Answer from the drawing. Dimensions are ordinates in mm from the lowest x, y and z of the part. Round coordinates to 2 decimals unless told otherwise and drop trailing zeros. Loops run counter-clockwise (first coordinate to the right, second up) from the corner with the lowest first, then second, coordinate; pieces in that order, holes last. Notation, with made-up numbers: (9, 87.5) - (18, 87.5) arc R13 cw to (18, 111.5) - close; hole circle Ø11 at (42.25, 68.5). An arc over 180 degrees is marked (long way). Return JSON: item names as keys, results as strings.
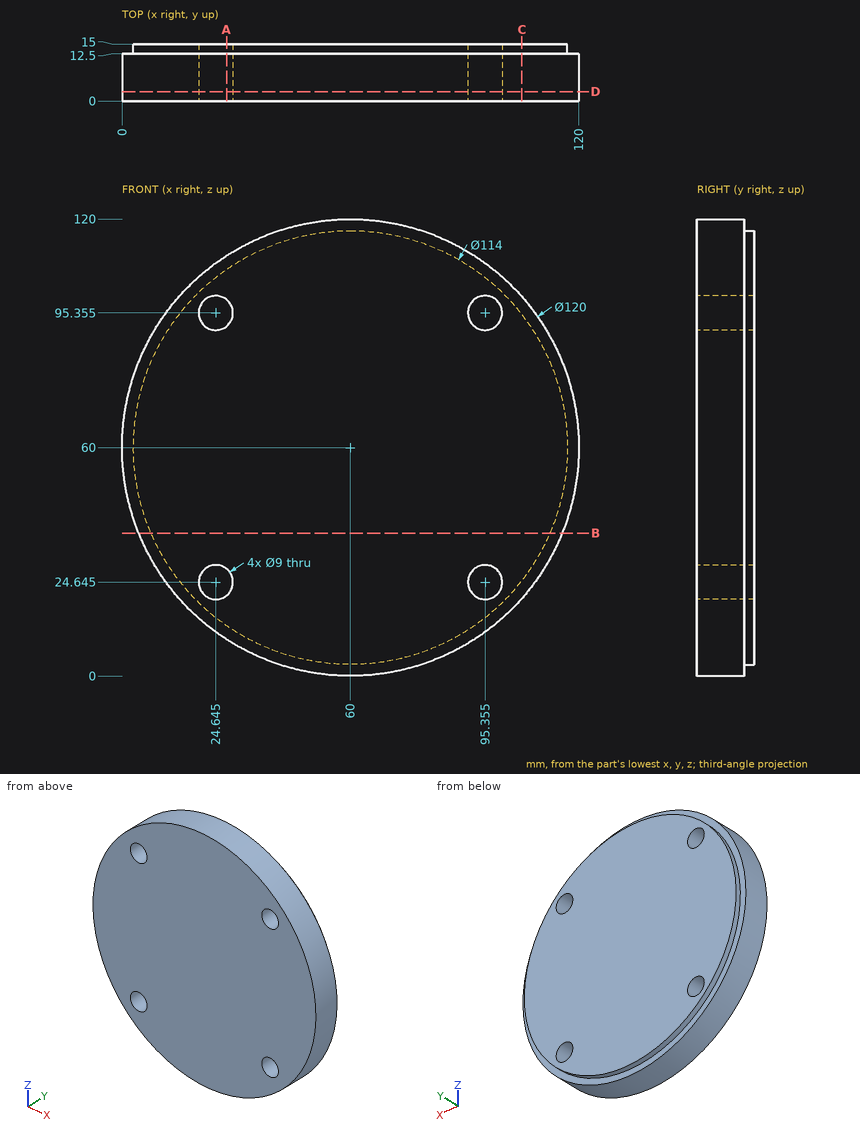
1) Flat-ended cylindrical pins translate along their axes: pin 1 (1 mm diameter, centred on y = 11.5, z = 104.5, fed in from +X); pin 2 (2 mm diameter, centred on x = 77.5, y = 11, fed in from -Z); pin 3 (5 mm diameter, centred on x = 16, y = 2, fed in from +Z). Find the tip coordinate at first contact, or state that the pin passes through.
Verdict:
{"pin 1": "stops at x = 100.79", "pin 2": "stops at z = 2.31", "pin 3": "stops at z = 103.33"}
2) Section C-C (x = 105) is taken. Give the vertices of the cut face in (y, z).
Verdict:
{"outline": "(0, 20.31) - (12.5, 20.31) - (12.5, 25.01) - (15, 25.01) - (15, 94.99) - (12.5, 94.99) - (12.5, 99.69) - (0, 99.69) - close"}
3) Section D-D (y = 2.5) is taken. Give the vertices of the cut face in (x, z) (1 decimal).
Verdict:
{"outline": "circle Ø120 at (60, 60); hole circle Ø9 at (24.6, 24.6); hole circle Ø9 at (24.6, 95.4); hole circle Ø9 at (95.4, 24.6); hole circle Ø9 at (95.4, 95.4)"}
4) Find the intervals of material crossed by L1, parallel to X at y = 3.75, z = 24.5; L2, parallel to X at y = 1.75, z = 25.5; L3, parallel to Y at x = 82, z = 6.5, in increasing order.
Verdict:
{"L1": "x = 11.63 to 20.15, 29.14 to 90.86, 99.85 to 108.37", "L2": "x = 10.91 to 20.23, 29.06 to 90.94, 99.77 to 109.09", "L3": "y = 0 to 12.5"}
5) Section B-B (z = 37.5) is taken. Give the vertices of the cut face in (x, y).
Verdict:
{"outline": "(4.38, 0) - (115.62, 0) - (115.62, 12.5) - (112.37, 12.5) - (112.37, 15) - (7.63, 15) - (7.63, 12.5) - (4.38, 12.5) - close"}
6) Section A-A (x = 27.5) is taken. Give the vertices of the cut face in (y, z) (1 decimal).
Verdict:
{"outline": "(0, 9.6) - (12.5, 9.6) - (12.5, 13.2) - (15, 13.2) - (15, 21.2) - (0, 21.2) - close; (0, 28.1) - (15, 28.1) - (15, 91.9) - (0, 91.9) - close; (0, 98.8) - (15, 98.8) - (15, 106.8) - (12.5, 106.8) - (12.5, 110.4) - (0, 110.4) - close"}
